Here's how the part is built. I have some questions about the finished solid (model axes, mm). A direction names the side the tool comes from. Coordinates: 2 decimals unless noted, no trailing zeros. Loops run counter-clockwise (first coordinate to the right, second up) from the corner with the lowest first, then second, coordinate; pieces in that order, holes last. Notation, with made-up numbers: (45.5, -39) -> (52.5, -39) arc R8 ccw to (52.5, -33) -> close; hole circle Ø1 at (85, 35.25). An arc over 180 degrees is marked (long way). Answer as a JSON object with one key per item and string values. Group by question number.
Q1. I want a section at D-D on z = 39. Write out the boundary of the cut face in (x, y).
Q2. I want a section at A-A on x = 0. Count the separate pieces of the cut face and the enclosed holes in it, then the cut area to 3 significant figures.
Q3. I want a section at C-C on z = 79. Write out the boundary of the cut face in (x, y) (1 decimal), then the cut area to 3 significant figures.
Q4. Thinking about a two-plate mould opening in X: for faces 3 (the cylindrical face through (16, -7, 81)), 4 (the cylindrical face through (0.148, 9.083, 6.163)), 5 (the cylindrical face through (-12.071, 1.042, 82.696)), 6 (the cylindrical face through (-2.986, -9.129, 11.078)), which applies, released by +X, released by -X, zero draft, split by the parting line, or undercut?
Q5. I'm going to push flat-ended pins straight in: pin 1 (8 mm diameter, centred on x = 8.5, z = 60.5, fed in from +Y); pin 2 (6 mm diameter, centred on x = 0, z = 44.5, fed in from +Y); pin 3 (4 mm diameter, centred on x = 0, z = 9.525, fed in from +Y); pin 4 (1 mm diameter, centred on x = 7.5, z = 38, fed in from -Y). Where does each tip first touch, or does it pass through?
Q6. I need wall thicknesses on line 1 (Z direction, x = 10, y = 1.5) (3 decimals); line 2 (X direction, y = 7, z = 47); line 3 (X direction, y = 5.5, z = 83). Which ranges of each line are inside material? Lowest first, please.
Q7. On a 3-axis mill with a long thin cutter (end or side, diameter ignored), from which of +Z, -Z, +X, -X, +Y, -Y can I reach the whole of each face in a straight line? I mean faces 1 (the cylindrical face through (7.8, 2.5, 45.1)), 2 (the cylindrical face through (11.917, 4.763, 80.489)). Say none if no direction works.
```python
from build123d import *

# Parameters (mm, degrees)
SKETCH1_R               = 10.7315
SKETCH1_R_2             = 8.1915
BOSS_EXTRUDE1_DEPTH     = 88.9
SKETCH4_R               = 17.4625
BOSS_EXTRUDE2_DEPTH     = 19.05
CUT_EXTRUDE1_DEPTH      = 93.266395901
CUT_EXTRUDE1_DEPTH_BACK = 93.266395901
SKETCH5_R               = 3.3655
CUT_EXTRUDE2_DEPTH      = 93.266396035
CUT_EXTRUDE2_DEPTH_BACK = 93.266396035
SKETCH7_R               = 3.3655
SKETCH8_R               = 8.1915
CUT_EXTRUDE3_DEPTH      = 93.266396035
BOSS_EXTRUDE3_START     = 3.175
SKETCH9_R               = 17.4625
BOSS_EXTRUDE3_DEPTH     = 3.175


with BuildPart() as part:
    # Sketch1 → Boss-Extrude1 (new body)
    with BuildSketch(Plane.XY):
        Circle(SKETCH1_R)
        Circle(SKETCH1_R_2, mode=Mode.SUBTRACT)
    extrude(amount=BOSS_EXTRUDE1_DEPTH)

    # Sketch4 → Boss-Extrude2 (add)
    with BuildSketch(Plane.XY.offset(88.9)):
        Circle(SKETCH4_R)
    extrude(amount=-BOSS_EXTRUDE2_DEPTH)

    # Sketch5 → Cut-Extrude1 (cut, two sides: drawn at the far end of the back side and taken through both)
    with BuildSketch(Plane(origin=(0, 0, 0), x_dir=(0, 0, -1), z_dir=(1, 0, 0)).offset(-CUT_EXTRUDE1_DEPTH_BACK)):
        with Locations(Location((-79.375, 1.5875, 0), (0, 0, 331.855418691))):
            Circle(SKETCH5_R)
    extrude(amount=CUT_EXTRUDE1_DEPTH + CUT_EXTRUDE1_DEPTH_BACK, mode=Mode.SUBTRACT)

    # Sketch7 → Cut-Extrude2 (cut, two sides: drawn at the far end of the back side and taken through both)
    with BuildSketch(Plane(origin=(0, 0, 0), x_dir=(1, 0, 0), z_dir=(0, 1, 0)).offset(-CUT_EXTRUDE2_DEPTH_BACK)):
        with Locations(Location((0, -9.525, 0), (0, 0, 270))):
            Circle(SKETCH7_R)
    extrude(amount=CUT_EXTRUDE2_DEPTH + CUT_EXTRUDE2_DEPTH_BACK, mode=Mode.SUBTRACT)

    # Sketch8 → Cut-Extrude3 (cut, through all)
    with BuildSketch(Plane.XY.offset(88.9)):
        Circle(SKETCH8_R)
    extrude(amount=-CUT_EXTRUDE3_DEPTH, mode=Mode.SUBTRACT)

    # Sketch9 → Boss-Extrude3 (add)
    with BuildSketch(Plane.XY.offset(88.9).offset(BOSS_EXTRUDE3_START)):
        Circle(SKETCH9_R)
    extrude(amount=-BOSS_EXTRUDE3_DEPTH)


solid = part.part
```
Result set:
{
 "1": {"outline": "circle Ø21.46 at (0, 0); hole circle Ø16.38 at (0, 0)"},
 "2": {"separate pieces": "3", "enclosed holes": "0", "area": "785 mm²"},
 "3": {"outline": "(-17.4, -1.8) arc R17.5 ccw to (17.4, -1.8) -> (8, -1.8) arc R8.2 cw to (-8, -1.8) -> close; (-16.8, 4.9) -> (-6.5, 4.9) arc R8.2 cw to (6.5, 4.9) -> (16.8, 4.9) arc R17.5 ccw to start", "area": "620 mm²"},
 "4": {"face 3": "split by the parting line", "face 4": "undercut", "face 5": "zero draft", "face 6": "undercut"},
 "5": {"pin 1": "stops at y = 9.74", "pin 2": "stops at y = 10.73", "pin 3": "passes through", "pin 4": "stops at y = -8.13"},
 "6": {"line 1": "z = 0 to 76.011, 82.739 to 92.075", "line 2": "x = -8.13 to -4.25, 4.25 to 8.13", "line 3": "x = -16.57 to -6.07, 6.07 to 16.57"},
 "7": {"face 1": "-Z", "face 2": "+X, -X"}
}
